Can you work these out from the model? Positions are in its coordinate system, mm. A direction names the side the tool comes from. Round coordinates to 2 decimals unless told otherwise and drop trailing zeros. Loops run counter-clockwise (first coordinate to the right, second up) from the corner with the lowest first, then second, coordinate; pieces in that order, holes last. Notation, with made-up numbers: (74, 32.5) -> (118, 32.5) arc R11 ccw to (118, 51.5) -> close; hole circle Ø1 at (60.5, -8). An arc over 180 degrees is marked (long way). Answer as a JSON object with one key per item and string values.
```python
from build123d import *

# Parameters (mm, degrees)
SKETCH1_W              = 21.5
SKETCH1_H              = 19
COMBINE_BASE_DEPTH     = 1
STAND_OFFS_DEPTH       = 2
PCB_CONTAINERS_DEPTH   = 1.5
SNAP_INS_DEPTH         = 1.15
INSIDE_FILLETS_R       = 1
OUTSIDE_FILLETS_R      = 2.7
CLICK_IN_CHAMFERS_SIZE = 0.5
PULL_OUT_CHAMFERS_SIZE = 0.5


with BuildPart() as part:
    # Sketch1 → Combine Base (new body)
    with BuildSketch(Plane(origin=(0, 0, 0), x_dir=(1, 0, 0), z_dir=(0, 1, 0))):
        Rectangle(SKETCH1_W, SKETCH1_H)
    extrude(amount=COMBINE_BASE_DEPTH)

    # Sketch4 → Stand offs (add)
    with BuildSketch(Plane(origin=(0, 1, 0), x_dir=(1, 0, 0), z_dir=(0, 1, 0))):
        Polygon((-10.75, 3.8), (-8.05, 3.8), (-8.05, 6.8), (-5.05, 6.8), (-5.05, 9.5), (-10.75, 9.5), align=None)
        Polygon((-8.05, -3.8), (-10.75, -3.8), (-10.75, -9.5), (-5.05, -9.5), (-5.05, -6.8), (-8.05, -6.8), align=None)
        Polygon((5.05, -6.8), (5.05, -9.5), (10.75, -9.5), (10.75, -3.8), (8.05, -3.8), (8.05, -6.8), align=None)
        Polygon((10.75, 9.5), (5.05, 9.5), (5.05, 6.8), (8.05, 6.8), (8.05, 3.8), (10.75, 3.8), align=None)
    extrude(amount=STAND_OFFS_DEPTH)

    # Sketch5 → PCB Containers (add)
    with BuildSketch(Plane(origin=(0, 3, 0), x_dir=(1, 0, 0), z_dir=(0, 1, 0))):
        Polygon((-10.75, 3.8), (-9.55, 3.8), (-9.55, 8.3), (-5.05, 8.3), (-5.05, 9.5), (-10.75, 9.5), align=None)
        Polygon((9.55, 8.3), (9.55, 3.8), (10.75, 3.8), (10.75, 9.5), (5.05, 9.5), (5.05, 8.3), align=None)
        Polygon((9.55, -8.3), (5.05, -8.3), (5.05, -9.5), (10.75, -9.5), (10.75, -3.8), (9.55, -3.8), align=None)
        Polygon((-10.75, -9.5), (-5.05, -9.5), (-5.05, -8.3), (-9.55, -8.3), (-9.55, -3.8), (-10.75, -3.8), align=None)
    extrude(amount=PCB_CONTAINERS_DEPTH)

    # Sketch6 → Snap Ins (add)
    with BuildSketch(Plane(origin=(0, 4.5, 0), x_dir=(1, 0, 0), z_dir=(0, 1, 0))):
        Polygon((-5.05, 7.8), (-5.05, 9.5), (-10.75, 9.5), (-10.75, 3.8), (-9.05, 3.8), (-9.05, 7.8), align=None)
        Polygon((-9.05, -3.8), (-10.75, -3.8), (-10.75, -9.5), (-5.05, -9.5), (-5.05, -7.8), (-9.05, -7.8), align=None)
        Polygon((10.75, -9.5), (10.75, -3.8), (9.05, -3.8), (9.05, -7.8), (5.05, -7.8), (5.05, -9.5), align=None)
        Polygon((10.75, 9.5), (5.05, 9.5), (5.05, 7.8), (9.05, 7.8), (9.05, 3.8), (10.75, 3.8), align=None)
    extrude(amount=SNAP_INS_DEPTH)

    # Inside Fillets
    inside_fillets_edges = [part.edges().sort_by_distance(p)[0] for p in [
        (9.55, 3.75, -8.3),
        (9.55, 3.75, 8.3),
        (-9.55, 3.75, 8.3),
        (-9.05, 5.075, 7.8),
        (9.05, 5.075, 7.8),
        (-8.05, 2, -6.8),
        (9.05, 5.075, -7.8),
        (-9.05, 5.075, -7.8),
        (-8.05, 2, 6.8),
        (8.05, 2, 6.8),
        (8.05, 2, -6.8),
        (-9.55, 3.75, -8.3),
    ]]
    fillet(inside_fillets_edges, radius=INSIDE_FILLETS_R)

    # Outside Fillets
    outside_fillets_edges = [part.edges().sort_by_distance(p)[0] for p in [
        (10.75, 2.825, 9.5),
        (-10.75, 2.825, 9.5),
        (-10.75, 2.825, -9.5),
        (10.75, 2.825, -9.5),
    ]]
    fillet(outside_fillets_edges, radius=OUTSIDE_FILLETS_R)

    # Click in Chamfers
    click_in_chamfers_edges = [part.edges().sort_by_distance(p)[0] for p in [
        (-9.05, 5.65, 5.3),
        (9.05, 5.65, 5.3),
        (6.55, 5.65, -7.8),
        (-9.05, 5.65, -5.3),
        (6.55, 5.65, 7.8),
        (-6.55, 5.65, 7.8),
        (-6.55, 5.65, -7.8),
        (9.05, 5.65, -5.3),
        (8.757106781, 5.65, 7.507106781),
        (-8.757106781, 5.65, 7.507106781),
        (-8.757106781, 5.65, -7.507106781),
        (8.757106781, 5.65, -7.507106781),
    ]]
    chamfer(click_in_chamfers_edges, length=CLICK_IN_CHAMFERS_SIZE)

    # Pull out Chamfers
    pull_out_chamfers_edges = [part.edges().sort_by_distance(p)[0] for p in [
        (-6.55, 4.5, -7.8),
        (-9.05, 4.5, -5.3),
        (-8.757106781, 4.5, -7.507106781),
        (9.05, 4.5, -5.3),
        (6.55, 4.5, -7.8),
        (8.757106781, 4.5, -7.507106781),
        (6.55, 4.5, 7.8),
        (9.05, 4.5, 5.3),
        (8.757106781, 4.5, 7.507106781),
        (-9.05, 4.5, 5.3),
        (-6.55, 4.5, 7.8),
        (-8.757106781, 4.5, 7.507106781),
    ]]
    chamfer(pull_out_chamfers_edges, length=PULL_OUT_CHAMFERS_SIZE - 0.0001)  # a hair under: the kernel refuses the full size


solid = part.part
```
Q1. I want a section at A-A, the plane y = 2.3. Give the number of separate pieces and of enclosed holes in the cut face, then the cut area to 3 significant figures.
Determined:
{"separate pieces": "4", "enclosed holes": "0", "area": "88.6 mm²"}
Q2. On a 3-axis mill with a long thin cutter (end or side, diameter ignored), from which of +Z, -Z, +X, -X, +Y, -Y can I reach the whole of each face in a straight line? I mean faces 3 (the flat face through (10, 3, 3.8)), 4 (the flat face through (-7, 4, -8.3)), 5 (the flat face through (5.05, 2.8, 8.4)). Say none if no direction works.
Determined:
{"face 3": "+X, -X, +Y", "face 4": "none", "face 5": "+Z, -Z, +Y"}
Q3. I'm going to push flat-ended pins straight in: pin 1 (2.5 mm diameter, centred on x = 8, z = 5, fed in from +Y); pin 2 (5.5 mm diameter, centred on x = 0, z = 0, fed in from +Y). Where does each tip first touch, or does it pass through?
Determined:
{"pin 1": "y = 5.35", "pin 2": "y = 1"}
Q4. If I drill on L1, parallel to X at y = 4.2, z = -6.5; L2, parallel to X at y = 2.1, z = 4.75; L3, parallel to Z at x = 6, y = 4.6, over which ranges is the centre line in solid material (lowest first)? Write a range as [from, to].
Determined:
{"L1": "[-10.75, -9.55], [9.55, 10.75]", "L2": "[-10.75, -8.05], [8.05, 10.75]", "L3": "[-9.5, -8.2], [8.2, 9.5]"}
Q5. We'd pull the mould along X, two halves only. Please class faces 1 (the flat face through (-6, 2, 6.8)), 2 (the flat face through (10, 3, -3.8)): pulls with the +X half, pulls with the -X half, needs draft (parallel to the pull), parting line crosses it, or undercut.
Determined:
{"face 1": "undercut", "face 2": "needs draft"}
Q6. I want a section at D-D, the plane z = 2.75. Write out the boundary of the cut face in (x, y), then the cut area to 3 significant figures.
Determined:
{"outline": "(-10.75, 0) -> (10.75, 0) -> (10.75, 1) -> (-10.75, 1) -> close", "area": "21.5 mm²"}
